Build history of the part. All positions in model axes, mm. A direction names the side the tool comes from. Round coordinates to 2 decimals unless told otherwise and drop trailing zeros. Write each loop counter-clockwise with the first axis right and the second up, starting at its lowest first coordinate (ties: lowest second). Pieces come first, ordered by that corner, then holes. Notation, with made-up numbers: (72, 49) -> (100, 49) arc R15 cw to (100, 70) -> close; hole circle Ø1 at (89, 57.5). An arc over 180 degrees is marked (long way). Answer in a Markdown table with one row per item. Add a question column.
Autodesk Inventor part; units mm, degrees
ref_plane "Work Plane1" through (-37.4166, 11.3496, -26) normal (0, 0, -1) x (0, 1, 0)
ref_plane "Work Plane2" through (-37.5, -28.6504, -144) normal (0, 0, -1) x (0, 1, 0)
ref_plane "Work Plane3" through (-7.5, 26.4496, -42.5) normal (0, 1, 0) x (0, 0, 1)
sketch "Sketch1" plane through (0, 0, 0) normal (0, 0, 1) x (1, 0, 0)
  arc A0 (-16, 36.5624) -> (16, 36.5624) centre (0, 8.8496) ccw
  line L0 (-16, 36.5624) -> (0, 45.8)
  line L1 (0, 45.8) -> (16, 36.5624)
  line L2 (37.5, 8.8496) -> (37.5, -28.6504)
  arc A1 (37.5, 8.8496) -> (-37.5, 8.8496) centre (0, 8.8496) ccw
  line L3 (-37.5, -28.6504) -> (-37.5, 8.8496)
  line L4 (37.5, -28.6504) -> (-37.5, -28.6504)
  line L5 (-37.5, -28.6504) -> (37.5, -28.6504)
  line L6 (37.5, -28.6504) -> (37.5, -48.6504)
  line L7 (37.5, -48.6504) -> (-37.5, -48.6504)
  line L8 (-37.5, -48.6504) -> (-37.5, -28.6504)
  point P0 (0, 0)
  dimension "d0" = 20
ref_plane "Work Plane1" through (-37.4166, 11.3496, -26) normal (0, 0, -1) x (0, 1, 0)
extrude "Extrusion1" add sketch "Sketch1" against normal up to surface (26 mm away) contours L0 L1 A0 | L2 L4 L3 A1 | L6 L7 L8 L4
sketch "Sketch2" plane through (0, 8.8496, -26) normal (0, 0, -1) x (-1, 0, 0)
  line L0 (-37.5, -57.5) -> (-37.5, 0)
  line L1 (37.5, -57.5) -> (-37.5, -57.5)
  line L2 (37.5, 0) -> (37.5, -57.5)
  line L3 (-37.5, -3.5) -> (-28.6182, -3.5)
  line L4 (-37.5, -57.5) -> (37.5, -57.5)
  line L5 (37.5, -57.5) -> (37.5, -3.5)
  line L6 (37.5, -3.5) -> (-37.5, -3.5)
  line L7 (-37.5, -3.5) -> (-37.5, -57.5)
  point P0 (0, -8.8496)
ref_plane "Work Plane2" through (-37.5, -28.6504, -144) normal (0, 0, -1) x (0, 1, 0)
extrude "Extrusion2" add sketch "Sketch2" along normal up to surface (118 mm away)
sketch "Sketch3" plane through (-37.5, 5.3496, -26) normal (0, 1, 0) x (1, 0, 0)
  line L0 (75, 118) -> (0, 118)
  line L1 (0, 0) -> (0, 118)
  line L2 (75, 0) -> (0, 0)
  line L3 (75, 0) -> (75, 118)
  line L4 (80, 0) -> (-5, 0)
  line L5 (-5, 0) -> (-5, 142)
  line L6 (-5, 142) -> (80, 142)
  line L7 (80, 142) -> (80, 0)
  line L8 (37.5, 0) -> (37.5, 165)
  arc A0 (72.5, 142) -> (2.5, 142) centre (37.5, 142) ccw construction
  arc A1 (80, 142) -> (45, 177) centre (45, 142) ccw
  arc A2 (30, 177) -> (-5, 142) centre (30, 142) ccw
  line L9 (45, 177) -> (30, 177)
  line L10 (64.25, 165) -> (10.75, 165)
  arc A3 (45.75, 200) -> (10.75, 165) centre (45.75, 165) ccw
  line L11 (45.75, 165) -> (45.75, 200) construction
  line L12 (45.75, 165) -> (10.75, 165) construction
  arc A4 (64.25, 165) -> (29.25, 200) centre (29.25, 165) ccw
  line L13 (29.25, 165) -> (29.25, 200) construction
  line L14 (29.25, 165) -> (64.25, 165) construction
  line L15 (46, 195.7317) -> (29, 195.7317)
  line L16 (37.5, 109) -> (97.5, 109) construction
  circle A5 centre (97.5, 109) radius 7.5 construction
  arc A6 (80, 56.5596) -> (105, 109) centre (37.5, 109) ccw construction
  line L17 (105, 109) -> (105, 74)
  arc A7 (80, 21.5596) -> (105, 74) centre (37.5, 74) ccw
  line L18 (97.5, 116.5) -> (80, 116.5)
  arc A8 (105, 109) -> (97.5, 116.5) centre (97.5, 109) ccw
  point P0 (37.5, -26)
  point P1 (37.5, 118)
  point P2 (37.5, 142)
  dimension "d5" = 5
  dimension "d6" = 5
  dimension "d7" = 24
  dimension "d8" = 35
  dimension "d9" = 35
  dimension "d10" = 35
  dimension "d11" = 47
  dimension "d12" = 53.5
  dimension "d13" = 90
  dimension "d14" = 90
  dimension "d15" = 35
  dimension "d16" = 35
  dimension "d17" = 17
  dimension "d26" = 15
  dimension "d27" = 60
  dimension "d28" = 109
  dimension "d29" = 35
ref_plane "Work Plane3" through (-7.5, 26.4496, -42.5) normal (0, 1, 0) x (0, 0, 1)
extrude "Extrusion3" add sketch "Sketch3" along normal up to surface (21.1 mm away) contours L3 L2 L8 L0 | L0 L8 L6 L7 L4 L3 | L8 L2 L1 L0 | L0 L1 L4 L5 L6 L8 | L8 L10 A4 A1 L6 | L6 A2 A3 L10 L8 | L10 A3 A2 L9 A1 A4 | L7 L18 A8 L17 A7 | A3 L15 A4 A1 L9 A2
ref_plane "Work Plane4" through (12.5, 5.3496, -168) normal (-1, 0, 0) x (0, 0, 1)
ref_plane "Work Plane6" through (0, -1.1504, 0) normal (0, -1, 0) x (1, 0, 0)
ref_plane "Work Plane5" through (0, 46.3496, 0) normal (0, -1, 0) x (1, 0, 0)
ref_plane "Work Plane7" through (0, 0, -110.8659) normal (0, 0, 1) x (1, 0, 0)
equation "\"d9\" = d8"
equation "\"d10\" = d8"
equation "\"d15\" = d8"
equation "\"d16\" = d8"
properties part number "Space Envelope"
(1) Saw through at B-B (z = -130). List the corners of the cut face in (x, y).
(2) Saw through at A-A (x = 0). List the corners of the cut face in (y, z).
(3) Drop flat-ended pins along their axis: P1, Ø9, axis at x = 54.5, y = 11.5, coming from the -Z side; P2, Ø1, axis at x = 15, z = -140.5, coming from the +Y side; P3, Ø1, axis at x = -30.5, y = -13.5, coming from the +Z side; P4, Ø10.5, axis at y = 12.5, z = -153, coming from the +X side. Give the stop position or say it passes through.
(4) Probe line 1 along X through (y, z) = (-34.5, -62); line 2 along Y through (x, z) = (-28, -153.5); line 3 along Z through (x, y) = (34.5, 1.5). List the from-to ranges inside material, lowest first.
(5) Saw through at C-C (y = 34). List the corners of the cut face in (x, z).
(6) Which spindle directions (+Z, -Z, +X, -X, +Y, -Y) get a long thin tool onto all of the face, cutting with end or side? Do faces 1 (the face through (39, 16, -26)), 2 (the face through (0.82, 46.34, -12.82)), 3 (the face through (51, 16, -142.5)), 4 (the face through (42.5, 16, -37)), 5 (the face through (0, 34, -26)). Say none if no direction does.
Answer sheet:
| question | item | result |
|---|---|---|
| 1 | outline | (-42.5, 5.35) -> (-37.5, 5.35) -> (-37.5, -48.65) -> (37.5, -48.65) -> (37.5, 5.35) -> (67.5, 5.35) -> (67.5, 26.45) -> (-42.5, 26.45) -> close |
| 2 | outline | (-48.65, -144) -> (5.35, -144) -> (5.35, -221.73) -> (26.45, -221.73) -> (26.45, -26) -> (46.35, -26) -> (46.35, 0) -> (-48.65, 0) -> close |
| 3 | P1 | stops at z = -142.5 |
| 3 | P2 | stops at y = 26.45 |
| 3 | P3 | stops at z = 0 |
| 3 | P4 | stops at x = 42.5 |
| 4 | line 1 | x = -37.5 to 37.5 |
| 4 | line 2 | y = 5.35 to 26.45 |
| 4 | line 3 | z = -144 to 0 |
| 5 | outline | (-27.82, -26) -> (27.82, -26) -> (27.82, 0) -> (-27.82, 0) -> close |
| 6 | face 1 | +Z, +X, +Y |
| 6 | face 2 | +Z, +Y |
| 6 | face 3 | -Z, +X, +Y, -Y |
| 6 | face 4 | +Z, +X, +Y, -Y |
| 6 | face 5 | -Z, +X, -X, +Y |
